from build123d import *

# Parameters (mm, degrees)
SKETCH1_R           = 16
SKETCH1_R_2         = 14
BOSS_EXTRUDE1_DEPTH = 590
SKETCH2_R           = 35
BOSS_EXTRUDE2_DEPTH = 3
CHAMFER1_SIZE       = 2
SKETCH4_R           = 3.25
CUT_EXTRUDE2_DEPTH  = 594


with BuildPart() as part:
    # Sketch1 → Boss-Extrude1 (new body)
    with BuildSketch(Plane(origin=(0, 0, 0), x_dir=(1, 0, 0), z_dir=(0, 1, 0))):
        Circle(SKETCH1_R)
        Circle(SKETCH1_R_2, mode=Mode.SUBTRACT)
    extrude(amount=BOSS_EXTRUDE1_DEPTH)

    # Sketch2 → Boss-Extrude2 (add)
    with BuildSketch(Plane(origin=(0, 590, 0), x_dir=(1, 0, 0), z_dir=(0, 1, 0))):
        Circle(SKETCH2_R)
    extrude(amount=BOSS_EXTRUDE2_DEPTH)

    # Chamfer1
    chamfer1_edges = [part.edges().sort_by_distance(p)[0] for p in [
        (-16, 590, 0),
    ]]
    chamfer(chamfer1_edges, length=CHAMFER1_SIZE)

    # Sketch4 → Cut-Extrude2 (cut, through all)
    with BuildSketch(Plane(origin=(0, 593, 0), x_dir=(1, 0, 0), z_dir=(0, 1, 0))):
        with Locations((0, 27.5)):
            Circle(SKETCH4_R)
        with Locations((26.154054198, 8.497967345)):
            Circle(SKETCH4_R)
        with Locations((16.164094438, -22.247967345)):
            Circle(SKETCH4_R)
        with Locations((-16.164094438, -22.247967345)):
            Circle(SKETCH4_R)
        with Locations((-26.154054198, 8.497967345)):
            Circle(SKETCH4_R)
    extrude(amount=-CUT_EXTRUDE2_DEPTH, mode=Mode.SUBTRACT)


solid = part.part
Verification items for the finished model (mm, model axes). A direction names the side the tool comes from. Coordinates: 2 decimals unless noted, no trailing zeros. Order: outer loops, then holes, each group sorted by start corner. A loop starts at its lowest first (then second) coordinate and runs counter-clockwise, first axis right, second up.
Item 1: Release check for a two-part mould opening along X. For faces 1 (the face through (-3.47, 289.88, 15.62)), 2 (the face through (0, 590, 0)), 3 (the face through (0, 593, 0)) record: +X half, -X half, draft (parallel to the pull), parting line (faces both ways), or undercut.
Filled in:
face 1: parting line
face 2: undercut
face 3: draft
Item 2: Material ranges on L1, parallel to Z at x = 0, y = 447; L2, parallel to X at y = 433.5, z = 8; L3, parallel to Y at x = 1, z = 24.5, recorded low to high.
Filled in:
L1: z = -16 to -14, 14 to 16
L2: x = -13.86 to -11.49, 11.49 to 13.86
L3: y = 590 to 593
Item 3: Section check A-A, the plane z = 0. Enter the section's corners in (x, y).
Filled in:
outline: (-35, 590) - (-18, 590) - (-16, 588) - (-16, 0) - (-14, 0) - (-14, 590) - (14, 590) - (14, 0) - (16, 0) - (16, 588) - (18, 590) - (35, 590) - (35, 593) - (-35, 593) - close
Item 4: Access from +Z, -Z, +X, -X, +Y, -Y to the whole of each face (thin tool, end or side, straight path). Record for faces 4 (the face through (15, 590, -16)), 5 (the face through (-28, 591, 21)).
Filled in:
face 4: -Y
face 5: +Y, -Y
Item 5: Section check B-B, the plane y = 341.5. Enter the section's corners in (x, z).
Filled in:
outline: circle Ø32 at (0, 0); hole circle Ø28 at (0, 0)
Item 6: Depth check by flat-ended pin: pin 1 (10.5 mm diameter, centred on x = -16.16, z = 22.25, fed in from -Y); pin 2 (4 mm diameter, centred on x = 2, y = 466.5, fed in from +Z); pin 3 (6 mm diameter, centred on y = 474.5, z = 1.5, fed in from -X). Enter the tip coordinate at first touch or a pass-through.
Filled in:
pin 1: stops at y = 590
pin 2: stops at z = 16
pin 3: stops at x = -16
